For this review, take the finished solid that the model builds, in its own axes (mm). Face numbers are marked on the shaded views. A direction names the side the tool comes from. Give positions to 0.01 mm unless a question says otherwise; leave off trailing zeros. Write each loop counter-clockwise with the first axis right and the second up, starting at its lowest first coordinate (ties: lowest second). Pieces come first, ordered by that corner, then holes.
Q1. Machinability: for the marked faces 1 and 2, which of the approach directions +Z, -Z, +X, -X, +Y, -Y give a long, thin tool a straight path to every point of the face, cutting with its end or side? Answer none if there is none.
Q2. Mouldability with a two-part tool opening along X and no side actions: class the marked faces 3, 4 and 5 as released by +X, released by -X, zero draft, split by the parting line, or undercut.
Q3. For line 1 (Z direction, x = 0, y = -4.5); line 2 (X direction, y = -19.5, z = 1.5); line 3 (Y direction, x = 12, z = 2), list the stretches that pass through material, from the lowest coordinate up.
Q4. We need section A-A (y = -6). Write out the cut boundary in (x, z).
Q5. Insertion check: P1, Ø0.8, axis at x = 0, y = -4, coming from the -Z side; P2, Ø5, axis at y = -2.5, z = -9.5, coming from the +X side; P3, Ø12.5, axis at x = 0.5, z = 8.5, coming from the +Y side. Each pin has a flat end and moves straight along its axis. Give the tip position at first contact, or say it passes through.
```python
from build123d import *

# Parameters (mm, degrees)
F0_R     = 22.25
F1_DEPTH = 10
F2_W     = 9.2
F2_H     = 32.5
F3_DEPTH = 11.5
F5_DEPTH = 10
F6_R     = 1
F7_T     = -1.75
F8_W     = 1
F8_H     = 4.1
F9_DEPTH = 10
F10_R    = 1


with BuildPart() as f1:
    # F0 (on Front) → F1 (new body)
    with BuildSketch(Plane.XZ):
        Circle(F0_R)
    extrude(amount=F1_DEPTH)

    # F2 (on face) → F3 (join)
    with BuildSketch(Plane.XZ.offset(10)):
        Rectangle(F2_W, F2_H)
    extrude(amount=F3_DEPTH)

    # F4 (on face) → F5 (cut)
    with BuildSketch(Plane.YZ.offset(4.6)):
        with BuildLine():
            Line((-21.5, 16.25), (-21.5, 0))
            add(Edge.make_bspline(
                [(-21.5, 0), (-21.5, 9.096233188), (-21.5, 16.25), (-15.75, 16.25)],
                knots=[0, 0, 0, 0, 17.2373141759, 17.2373141759, 17.2373141759, 17.2373141759], degree=3))
            Line((-15.75, 16.25), (-21.5, 16.25))
        make_face()
        with BuildLine():
            add(Edge.make_bspline(
                [(-21.5, 0), (-21.5, -9.096233188), (-21.5, -16.25), (-15.75, -16.25)],
                knots=[0, 0, 0, 0, 17.2373141759, 17.2373141759, 17.2373141759, 17.2373141759], degree=3))
            Line((-21.5, 0), (-21.5, -16.25))
            Line((-21.5, -16.25), (-15.75, -16.25))
        make_face()
    extrude(amount=-F5_DEPTH, mode=Mode.SUBTRACT)

    # F6
    f6_edges = [f1.edges().sort_by_distance(p)[0] for p in [
        (4.6, -12.875, -16.25),
        (-4.6, -21.14469, -9.555694),
    ]]
    fillet(f6_edges, radius=F6_R)

    # F7
    f7_openings = [f1.faces().sort_by_distance(p)[0] for p in [
        (0, 0, 0),
    ]]
    offset(amount=F7_T, openings=f7_openings, kind=Kind.INTERSECTION)

    # F8 (on Front) → F9 (join)
    with BuildSketch(Plane.XZ):
        with Locations((0, 18.524242565)):
            Rectangle(F8_W, F8_H)
    extrude(amount=F9_DEPTH)

    # F10
    f10_edges = [f1.edges().sort_by_distance(p)[0] for p in [
        (-22.25, -10, 0),
    ]]
    fillet(f10_edges, radius=F10_R)


solid = f1.part
```
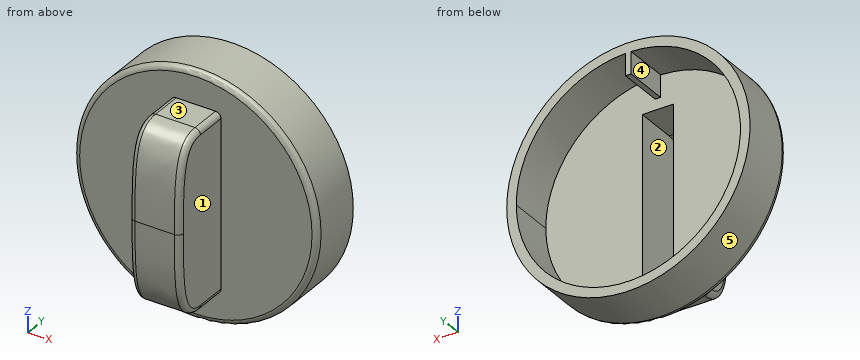
Computed:
1. face 1: +Z, -Z, +X, -Y
1. face 2: +Y
2. face 3: zero draft
2. face 4: undercut
2. face 5: split by the parting line
3. line 1: z = -22.25 to -20.5, 16.47 to 22.25
3. line 2: x = -4.6 to -2.85, 2.85 to 4.6
3. line 3: y = -10 to -8.25
4. outline: circle Ø44.5 at (0, 0); hole (-0.5, 16.47) - (-0.5, 20.49) arc R20.5 ccw (long way) to (0.5, 20.49) - (0.5, 16.47) - close
5. P1: stops at z = -22.25
5. P2: stops at x = 21.12
5. P3: stops at y = -8.25
